Geometry: final body of the model. Coordinates: model frame, mm. Face numbers are marked on the shaded views. A direction names the side the tool comes from. Give positions to 0.01 mm unless a question says otherwise; leave off trailing zeros. Write each loop counter-clockwise with the first axis right and the second up, starting at its lowest first coordinate (ties: lowest second). Pieces come first, ordered by that corner, then holes. Notation, with made-up numbers: (8.5, 23) - (55.5, 23) arc R21 cw to (55.5, 33) - close; hole circle Ø3 at (-8, -18.5). An arc over 180 degrees is marked (long way). One line per question, with ' | ' between items. Start each with the question number.
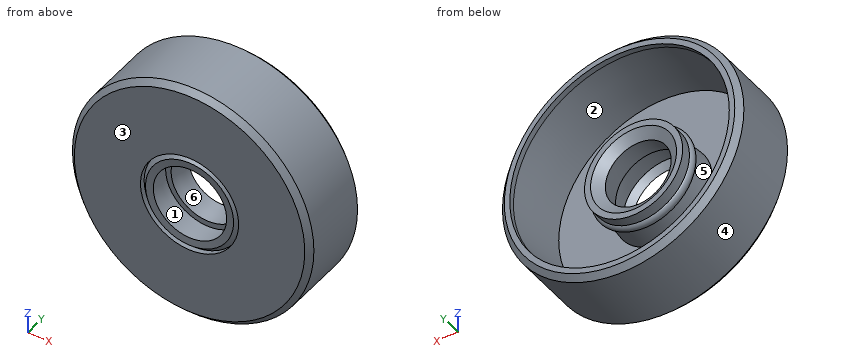
```python
from build123d import *


with BuildPart() as part:
    # 草图1 → 旋转1 (revolve)
    with BuildSketch(Plane.XY):
        with BuildLine():
            Line((-10.5, 0), (-4.473202091, 0))
            Line((-4.473202091, 0), (-4.473202091, 0.5))
            Line((-4.473202091, 0.5), (-4.015036504, 0))
            Line((-4.015036504, 0), (-3.340059177, 0.059052864))
            Line((-3.340059177, 0.059052864), (-4.015036504, 0.5))
            Line((-4.015036504, 0.5), (-3.840059177, 2.5))
            Line((-3.840059177, 2.5), (-3.340059177, 2.5))
            Line((-3.340059177, 2.5), (-3, 4.428571429))
            Line((-3, 4.428571429), (-3.918095147, 5.071428571))
            Line((-3.918095147, 5.071428571), (-4.473202091, 5.071428571))
            Line((-4.473202091, 5.071428571), (-4.473202091, 4.133224056))
            ThreePointArc((-4.473202091, 4.133224056), (-4.708452271, 3.630475426), (-4.273202091, 3.286010461))
            Line((-4.273202091, 3.286010461), (-4.473202091, 1))
            Line((-4.473202091, 1), (-9.518812351, 1))
            Line((-9.518812351, 1), (-10, 6.5))
            Line((-10, 6.5), (-10, 7))
            Line((-10, 7), (-10.5, 7))
            Line((-10.5, 7), (-11, 6.5))
            Line((-11, 6.5), (-11, 0.5))
            Line((-11, 0.5), (-10.5, 0))
        make_face()
    revolve(axis=Axis((0, 5.977335763, 0), (0, -1, 0)))


solid = part.part
```
1) Section A-A, the plane y = 1.75. Output: boundary loops of the cut face in (x, z), plus the area to 3 significant figures.
2) Line query: L1, parallel to X at y = 4.75, z = 1.25 (3 decimals); L2, parallel to Z at x = 0, y = 0.3; L3, parallel to Z at x = 0, y = 0.15. Output: solid intervals per line, ascending.
3) Section B-B, the plane y = 6. Output: boundary loops of the cut face in (x, z).
4) Pull-direction query (Z, two-part tool) for the marked faces 3, 4, 5 and 6; classes: +Z half, -Z half, draft (parallel to the pull), parting line (faces both ways), or undercut.
5) Reachability of the marked faces 1 and 2 from +Z, -Z, +X, -X, +Y, -Y: full face, straight path, thin tool, end or side. Return the list, or none.
6) First-contact query: pin 1 Ø6 at (x, z) = (-0.5, 2) entering from -Y; pin 2 Ø1.5 at (x, y) = (1, 6) entering from -Z; pin 3 Ø1 at (y, z) = (4.5, -3) entering from +X; pin 4 Ø2.5 at (x, z) = (-2, 1.5) entering from +Y. Flat tips, straight axial feed; report the tip coordinate or a pass-through.
Answer key:
1) outline: circle Ø22 at (0, 0); circle Ø8.82 at (0, 0); hole circle Ø19.17 at (0, 0); hole circle Ø7.81 at (0, 0) | area: 105 mm^2
2) L1: -10.929 to -9.767, -4.295 to -3.225, 3.225 to 4.295, 9.767 to 10.929 | L2: -10.8 to -4.47, -4.29 to -3.71, 3.71 to 4.29, 4.47 to 10.8 | L3: -10.65 to -4.47, -4.15 to -3.48, 3.48 to 4.15, 4.47 to 10.65
3) outline: circle Ø22 at (0, 0); hole circle Ø19.91 at (0, 0)
4) face 3: draft | face 4: parting line | face 5: undercut | face 6: undercut
5) face 1: none | face 2: +Y
6) pin 1: y = 0 | pin 2: z = -11 | pin 3: x = 10.71 | pin 4: y = 4.95
